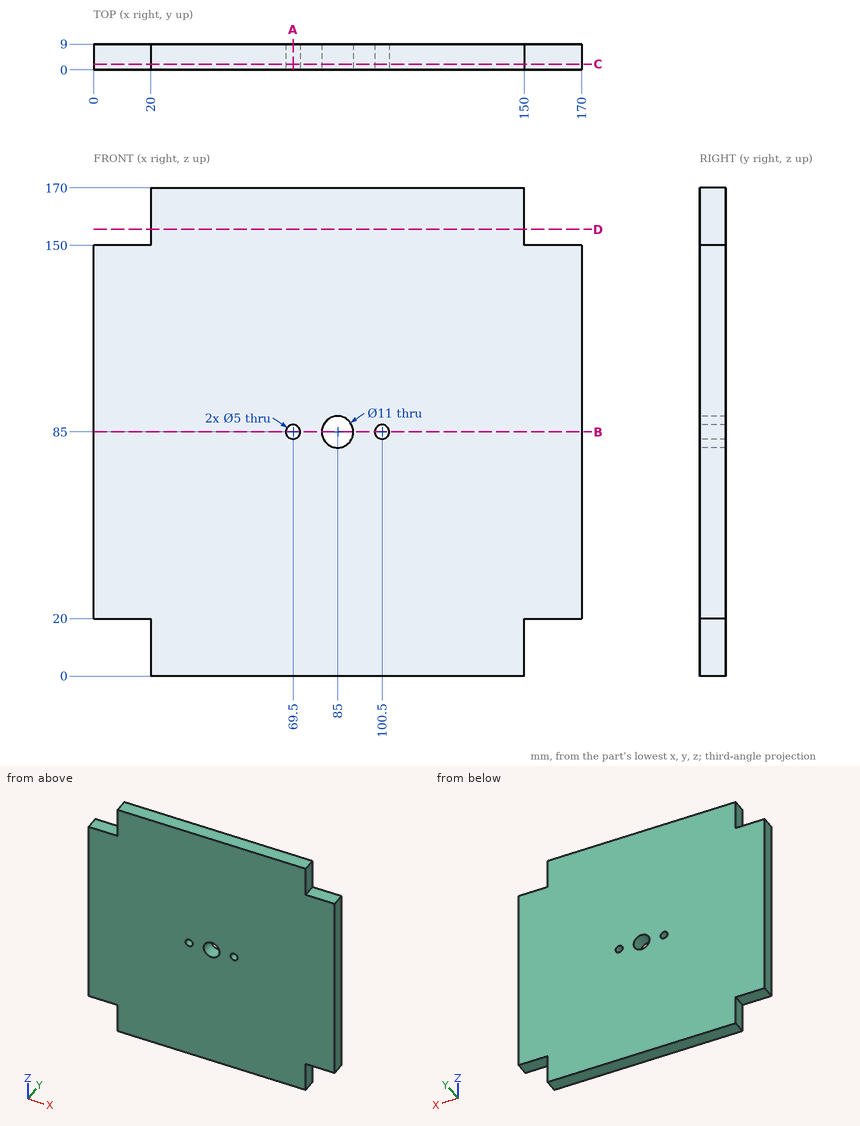
Answer from the drawing. Dimensions are ordinates in mm from the lowest x, y and z of the part. Coordinates: 2 decimals unless noted, no trailing zeros. Write each loop counter-clockwise with the first axis right and the second up, starting at its lowest first coordinate (ties: lowest second). Pieces come first, ordered by that corner, then holes. Notation, with made-up numbers: (12.25, -1) - (29.25, -1) arc R34 ccw to (29.25, 38) - close; hole circle Ø5 at (53, 41). An arc over 180 degrees is marked (long way). Return JSON: item names as keys, results as strings. Group by question number.
Q1. Flat-ended cylindrical pins translate along their axes: pin 1 Ø4.5 at (y, z) = (4.5, 11) entering from -X; pin 2 Ø4.5 at (x, y) = (15, 6.5) entering from -Z. Find the tip coordinate at first contact, or state that the pin passes through.
Q2. The part is cut by section D-D on z = 155.5. Write down the section's boundary in (x, y), and give its area (3 significant figures).
Q3. Find the intervals of material crossed by line 1 along X through (y, z) = (2.75, 85); line 2 along Z through (x, y) = (85, 5.5); line 3 along Z through (x, y) = (100.5, 4), in increasing order. Write a range as [from, to].
Q4. The part is cut by section A-A on x = 69.5. Write down the section's boundary in (y, z).
Q5. The part is cut by section C-C on y = 2. Write down the section's boundary in (x, z), and give its area (3 significant figures).
Q6. The part is cut by section B-B on z = 85. Write down the section's boundary in (x, y), and give its area (3 significant figures).
Evaluation:
{
 "1": {"pin 1": "stops at x = 20", "pin 2": "stops at z = 20"},
 "2": {"outline": "(20, 0) - (150, 0) - (150, 9) - (20, 9) - close", "area": "1,170 mm2"},
 "3": {"line 1": "x = [0, 67], [72, 79.5], [90.5, 98], [103, 170]", "line 2": "z = [0, 79.5], [90.5, 170]", "line 3": "z = [0, 82.5], [87.5, 170]"},
 "4": {"outline": "(0, 0) - (9, 0) - (9, 82.5) - (0, 82.5) - close; (0, 87.5) - (9, 87.5) - (9, 170) - (0, 170) - close"},
 "5": {"outline": "(0, 20) - (20, 20) - (20, 0) - (150, 0) - (150, 20) - (170, 20) - (170, 150) - (150, 150) - (150, 170) - (20, 170) - (20, 150) - (0, 150) - close; hole circle Ø5 at (69.5, 85); hole circle Ø11 at (85, 85); hole circle Ø5 at (100.5, 85)", "area": "27,200 mm2"},
 "6": {"outline": "(0, 0) - (67, 0) - (67, 9) - (0, 9) - close; (72, 0) - (79.5, 0) - (79.5, 9) - (72, 9) - close; (90.5, 0) - (98, 0) - (98, 9) - (90.5, 9) - close; (103, 0) - (170, 0) - (170, 9) - (103, 9) - close", "area": "1,340 mm2"}
}
